Can you work these out from the model? Positions are in its coordinate system, mm. A direction names the side the tool comes from. Give positions to 0.01 mm unless a question says otherwise; leave off trailing zeros. Loops run counter-clockwise (first coordinate to the right, second up) from the corner with the lowest first, then second, coordinate; pieces in that order, holes last. Notation, with made-up numbers: (60.5, -1) - (68.5, -1) arc R15 cw to (68.5, 20) - close; hole circle Ø8 at (45, 82). An arc over 180 degrees is marked (long way). Write item = value, one per line.
from build123d import *

# Parameters (mm, degrees)
HOLE_WIZARD_M31_D           = 3.4
HOLE_WIZARD_M31_CBORE_D     = 6.5
HOLE_WIZARD_M31_CBORE_DEPTH = 3
M3X0_51_D                   = 2.5
M3X0_51_DEPTH               = 15
M3X0_51_TIP                 = 0.751075774
CHAMFER_1_SIZE              = 0.5


with BuildPart() as part:
    # Эскиз2 → Повернуть1 (revolve)
    with BuildSketch(Plane(origin=(0, 0, 0), x_dir=(0, 0, -1), z_dir=(1, 0, 0))):
        Polygon((0, 0), (0, 16.5), (5, 16.5), (5, 6.3), (49, 6.3), (49, 0), align=None)
    revolve(axis=Axis((0, 0, -49), (0, 0, 1)))

    # Цековка для винта с внутренним шестигранником M31 (through all)
    with Locations(Plane.XY):
        with Locations((-12.5, 0), (0, 12.5), (12.5, 0), (0, -12.5)):
            CounterBoreHole(HOLE_WIZARD_M31_D / 2, HOLE_WIZARD_M31_CBORE_D / 2, HOLE_WIZARD_M31_CBORE_DEPTH)

    # Отверстие обработанное метчиком M3x0.51
    with Locations(Plane(origin=(2.706733298, -7.232806727, -49), x_dir=(-0.635524995, -0.772080294, 0), z_dir=(0, 0, -1))):
        with Locations((-3.864110878, 6.686444901)):
            Hole(M3X0_51_D / 2, depth=M3X0_51_DEPTH)
            with Locations((0, 0, -(M3X0_51_DEPTH + M3X0_51_TIP / 2))):  # 118° drill point
                Cone(0, M3X0_51_D / 2, M3X0_51_TIP, mode=Mode.SUBTRACT)

    # Фаска1
    chamfer_1_edges = [part.edges().sort_by_distance(p)[0] for p in [
        (0, -6.3, -49),
        (0, -16.5, 0),
    ]]
    chamfer(chamfer_1_edges, length=CHAMFER_1_SIZE)


solid = part.part
Q1. For pin 1 (5 mm diameter, centred on x = 12.5, y = 0, fed in from +Z); pin 2 (5 mm diameter, centred on x = 0, y = 12.5, fed in from -Z); pin 3 (1.5 mm diameter, centred on x = -5, z = -9, fed in from -Y), each with a flat end and sliding along its axis, tell me the tip position at first contact or that it passes through.
Output:
pin_1 = -3
pin_2 = -5
pin_3 = -4.65
Q2. We'd pull the mould along Y, two halves only. Please class faces 3 (the cylindrical face through (-0.423, 15.722, -1.479)), 4 (the cylindrical face through (3.83, -5, -27.05)), 5 (the flat face through (0, 0, 0)), 6 (the cylindrical face through (-0.423, -9.278, -1.479)): released by +Y, released by -Y, zero draft, split by the parting line, or undercut.
Output:
face_3 = undercut
face_4 = split by the parting line
face_5 = zero draft
face_6 = undercut
Q3. I need wall thicknesses on L1, parallel to Y at x = 0, z = -4; L2, parallel to X at y = 0, z = -43.75; L3, parallel to Z at x = 9, y = -10. Which ranges of each line are inside material? Lowest first, please.
Output:
L1 = -16.5 to -14.2, -10.8 to 10.8, 14.2 to 16.5
L2 = -6.3 to -1.25, 1.25 to 6.3
L3 = -5 to 0
Q4. Which directions (+Z, -Z, +X, -X, +Y, -Y) give clear straight access to the entire face, cutting with the end or side of a thin tool? Please do faces 1 (the cylindrical face through (-15.747, 0.143, -1.479)), 2 (the cylindrical face through (10.93, -0.65, -4.01)).
Output:
face_1 = +Z
face_2 = +Z, -Z
Q5. Imagine slicing it at B-B, the plane z = -40. Write out the boundary of the cut face in (x, y), then the cut area to 3 significant figures.
Output:
outline = circle Ø12.6 at (0, 0); hole circle Ø2.5 at (0, 0)
area = 120 mm2
Q6. Imagine slicing it at A-A, the plane z = -17. Write out the boundary of the cut face in (x, y).
Output:
outline = circle Ø12.6 at (0, 0)
